from build123d import *

# Parameters (mm, degrees)
SKETCH_W     = 60
SKETCH_H     = 10
SKETCH_R     = 1.55
SKETCH_R_2   = 1.6
SKETCH_R_3   = 1.65
SKETCH_R_4   = 1.7
SKETCH_R_5   = 1.75
PAD_DEPTH    = 10
SKETCH001_W  = 1
SKETCH001_H  = 6
PAD001_DEPTH = 1


with BuildPart() as part:
    # Sketch → Pad (new body)
    with BuildSketch(Plane.XY):
        Rectangle(SKETCH_W, SKETCH_H)
        with Locations((-20, 0)):
            Circle(SKETCH_R, mode=Mode.SUBTRACT)
        with Locations((-10, 0)):
            Circle(SKETCH_R_2, mode=Mode.SUBTRACT)
        Circle(SKETCH_R_3, mode=Mode.SUBTRACT)
        with Locations((10, 0)):
            Circle(SKETCH_R_4, mode=Mode.SUBTRACT)
        with Locations((20, 0)):
            Circle(SKETCH_R_5, mode=Mode.SUBTRACT)
    extrude(amount=PAD_DEPTH)

    # Sketch001 → Pad001 (join)
    with BuildSketch(Plane.XY.offset(10)):
        with Locations((-27.5, 0)):
            Rectangle(SKETCH001_W, SKETCH001_H)
        Polygon((25, 3), (28, 3), (28, 2), (26, 2), (26, 1), (28, 1), (28, -3), (24.966125, -3), (24.966125, -2), (27, -2), (27, 0), (25, 0), align=None)
    extrude(amount=PAD001_DEPTH)


solid = part.part
Work out the finished part from the listing and answer in its coordinate system (mm). A direction names the side the tool comes from. Coordinates: 2 decimals unless noted, no trailing zeros. Order: outer loops, then holes, each group sorted by start corner. A loop starts at its lowest first (then second) coordinate and runs counter-clockwise, first axis right, second up. Notation, with made-up numbers: (46.25, 31.5) - (85.25, 31.5) arc R17 cw to (85.25, 45.5) - close; hole circle Ø8 at (38.25, -34). An arc over 180 degrees is marked (long way). Put each result on its own line as item: value. Start each with the question number.
1) Find the intervals of material crossed by line 1 (Y direction, x = -10, z = 5); line 2 (X direction, y = 0.25, z = 6); line 3 (Y direction, x = 20, z = 2), in increasing order. Write a range as from..to.
2) Find section C-C (x = -20). Give the vertices of the cut face in (y, z).
3) Find section A-A (x = 10). Give the vertices of the cut face in (y, z), plus the area to 3 significant figures.
4) Find section B-B (z = 1). Give the vertices of the cut face in (x, y).
5) For faces 4 (the flat face through (28, -1, 10.5)), 5 (the flat face through (-27.5, 3, 10.5)), 6 (the flat face through (27, 1, 10.5)), determine the directions among +Z, -Z, +X, -X, +Y, -Y from which every point of the face is accessible in a straight line to the end or side of a thin tool.
6) Flat-ended cylindrical pins translate along their axes: pin 1 (5 mm diameter, centred on x = -16.5, y = 3, fed in from +Z); pin 2 (0.8 mm diameter, centred on y = -1.5, z = 10.5, fed in from -X); pin 3 (0.5 mm diameter, centred on y = 1.5, z = 10.5, fed in from +X). Find the tip coordinate at first contact, or state that the pin passes through.
7) For a pull along Y with two mould halves and no side action, classify faces 1 (the flat face through (26.5, 0.7, 11)), 2 (the flat face through (26.5, 3, 10.5)), 3 (the flat face through (27, 2, 10.5)) as released by +Y, released by -Y, zero draft, split by the parting line, or undercut.
Results list:
1. line 1: y = -5..-1.6, 1.6..5
1. line 2: x = -30..-21.53, -18.47..-11.58, -8.42..-1.63, 1.63..8.32, 11.68..18.27, 21.73..30
1. line 3: y = -5..-1.75, 1.75..5
2. outline: (-5, 0) - (-1.55, 0) - (-1.55, 10) - (-5, 10) - close; (1.55, 0) - (5, 0) - (5, 10) - (1.55, 10) - close
3. outline: (-5, 0) - (-1.7, 0) - (-1.7, 10) - (-5, 10) - close; (1.7, 0) - (5, 0) - (5, 10) - (1.7, 10) - close
3. area: 66.0 mm^2
4. outline: (-30, -5) - (30, -5) - (30, 5) - (-30, 5) - close; hole circle Ø3.1 at (-20, 0); hole circle Ø3.2 at (-10, 0); hole circle Ø3.3 at (0, 0); hole circle Ø3.4 at (10, 0); hole circle Ø3.5 at (20, 0)
5. face 4: +Z, +X, +Y, -Y
5. face 5: +Z, +X, -X, +Y
5. face 6: +Z, +X
6. pin 1: stops at z = 10
6. pin 2: stops at x = -28
6. pin 3: stops at x = 26
7. face 1: zero draft
7. face 2: released by +Y
7. face 3: undercut
